Verification items for the finished model (mm, model axes). A direction names the side the tool comes from. Round coordinates to 2 decimals unless told otherwise and drop trailing zeros. Order: outer loops, then holes, each group sorted by start corner. A loop starts at its lowest first (then second) coordinate and runs counter-clockwise, first axis right, second up. Notation, with made-up numbers: (41.25, 32) -> (62.25, 32) arc R9 cw to (62.25, 39) -> close; hole circle Ø11 at (27, -32). An arc over 180 degrees is marked (long way). Put each result on its own line as item: value.
from build123d import *

# Parameters (mm, degrees)
BOSS_EXTRUDE2_DEPTH       = 8.5
BOSS_EXTRUDE2_DEPTH_BACK  = 8.5
M6_TAPPED_HOLE1_D         = 5
M3X0_5_TAPPED_HOLE1_D     = 2.5
M3X0_5_TAPPED_HOLE1_DEPTH = 7.5
M3X0_5_TAPPED_HOLE1_TIP   = 0.751075774


with BuildPart() as part:
    # Model → Boss-Extrude2 (new, two sides: drawn at the far end of the back side and taken through both)
    with BuildSketch(Plane.XY.offset(-BOSS_EXTRUDE2_DEPTH_BACK)):
        with BuildLine():
            Line((64.292892272, 21.792891862), (67.207107272, 24.707105862))
            ThreePointArc((67.207107272, 24.707105862), (67.423880138, 25.031529799), (67.500000272, 25.414213862))
            Line((67.500000272, 25.414213862), (67.500000272, 34.5857853))
            ThreePointArc((67.500000272, 34.5857853), (67.423879863, 34.968468589), (67.207107272, 35.292891862))
            Line((67.207107272, 35.292891862), (64.292892272, 38.207106862))
            ThreePointArc((64.292892272, 38.207106862), (63.96846972, 38.423879155), (63.585787272, 38.499999862))
            Line((63.585787272, 38.499999862), (62.500000272, 38.499999862))
            ThreePointArc((62.500000272, 38.499999862), (61.79289349, 38.207106644), (61.500000272, 37.499999862))
            Line((61.500000272, 37.499999862), (61.500000272, 34.899999862))
            Line((61.500000272, 34.899999862), (58.500000272, 34.899999862))
            Line((58.500000272, 34.899999862), (58.500000272, 25.099999862))
            Line((58.500000272, 25.099999862), (61.500000272, 25.099999862))
            Line((61.500000272, 25.099999862), (61.500000272, 22.499999862))
            ThreePointArc((61.500000272, 22.499999862), (61.79289349, 21.792893081), (62.500000272, 21.499999862))
            Line((62.500000272, 21.499999862), (63.585787272, 21.499999862))
            ThreePointArc((63.585787272, 21.499999862), (63.968469605, 21.576120108), (64.292892272, 21.792891862))
        make_face()
    extrude(amount=BOSS_EXTRUDE2_DEPTH + BOSS_EXTRUDE2_DEPTH_BACK)

    # M6 Tapped Hole1 (through all)
    with Locations(Plane.ZY.offset(-58.500000272)):
        with Locations((0, 29.999999862)):
            Hole(M6_TAPPED_HOLE1_D / 2)

    # M3x0.5 Tapped Hole1
    with Locations(Plane(origin=(0, 0, -8.5), x_dir=(-1, 0, 0), z_dir=(0, 0, -1))):
        with Locations((-64.461940205, 29.965764831)):
            Hole(M3X0_5_TAPPED_HOLE1_D / 2, depth=M3X0_5_TAPPED_HOLE1_DEPTH)
            with Locations((0, 0, -(M3X0_5_TAPPED_HOLE1_DEPTH + M3X0_5_TAPPED_HOLE1_TIP / 2))):  # 118° drill point
                Cone(0, M3X0_5_TAPPED_HOLE1_D / 2, M3X0_5_TAPPED_HOLE1_TIP, mode=Mode.SUBTRACT)


solid = part.part
Item 1: Tool access check on faces 4 (the flat face through (61.5, 24, 0)), 5 (the flat face through (65.8, 36.7, -0.1)), 6 (the flat face through (61.5, 36, 0)). Record the directions out of +Z, -Z, +X, -X, +Y, -Y that give a thin tool (end or side, any length) a straight path to the whole face; none if there is none.
Check sheet entries:
face 4: +Z, -Z, -X, -Y
face 5: +Z, -Z, +X, +Y
face 6: +Z, -Z, -X, +Y
Item 2: Gauge pin test, flat ends, axial feed: pin 1 Ø1.5 at (x, z) = (66.5, 5) entering from -Y; pin 2 Ø1.5 at (x, z) = (59.5, 1.5) entering from -Y; pin 3 Ø1.3 at (y, z) = (36.5, -0.5) entering from -X; pin 4 Ø3 at (y, z) = (30, 0) entering from -X. Record the tip position at first contact, or that the pin passes through.
Check sheet entries:
pin 1: stops at y = 23.25
pin 2: stops at y = 25.1
pin 3: stops at x = 61.5
pin 4: passes through
Item 3: Section check D-D on z = 4.75. Record the boundary of the cut face in (x, y), then the cut area to 3 significant figures.
Check sheet entries:
outline: (58.5, 25.1) -> (61.5, 25.1) -> (61.5, 22.5) arc R1 ccw to (62.5, 21.5) -> (63.59, 21.5) arc R1 ccw to (64.29, 21.79) -> (67.21, 24.71) arc R1 ccw to (67.5, 25.41) -> (67.5, 34.59) arc R1 ccw to (67.21, 35.29) -> (64.29, 38.21) arc R1 ccw to (63.59, 38.5) -> (62.5, 38.5) arc R1 ccw to (61.5, 37.5) -> (61.5, 34.9) -> (58.5, 34.9) -> close
area: 119 mm^2
Item 4: Release check for a two-part mould opening along Y. For faces 1 (the cylindrical face through (64.191, 28.745, -5.278)), 2 (the flat face through (65.7, 23.2, -0.1)), 3 (the flat face through (58.5, 32, -2)) record: +Y half, -Y half, draft (parallel to the pull), parting line (faces both ways), or undercut.
Check sheet entries:
face 1: undercut
face 2: -Y half
face 3: draft
Item 5: Section check C-C on x = 62.75. Record the boundary of the cut face in (y, z), then the cut area to 3 significant figures.
Check sheet entries:
outline: (21.5, -8.5) -> (38.5, -8.5) -> (38.5, 8.5) -> (21.5, 8.5) -> close; hole circle Ø5 at (30, 0)
area: 269 mm^2
Item 6: Section check A-A on z = 0. Record the boundary of the cut face in (x, y), then the cut area to 3 significant figures.
Check sheet entries:
outline: (58.5, 25.1) -> (61.5, 25.1) -> (61.5, 22.5) arc R1 ccw to (62.5, 21.5) -> (63.59, 21.5) arc R1 ccw to (64.29, 21.79) -> (67.21, 24.71) arc R1 ccw to (67.5, 25.41) -> (67.5, 27.5) -> (58.5, 27.5) -> close; (58.5, 32.5) -> (67.5, 32.5) -> (67.5, 34.59) arc R1 ccw to (67.21, 35.29) -> (64.29, 38.21) arc R1 ccw to (63.59, 38.5) -> (62.5, 38.5) arc R1 ccw to (61.5, 37.5) -> (61.5, 34.9) -> (58.5, 34.9) -> close
area: 73.6 mm^2
Item 7: Section check B-B on y = 31.5. Record the boundary of the cut face in (x, z).
Check sheet entries:
outline: (58.5, -8.5) -> (67.5, -8.5) -> (67.5, -2) -> (58.5, -2) -> close; (58.5, 2) -> (67.5, 2) -> (67.5, 8.5) -> (58.5, 8.5) -> close
Item 8: Material ranges on L1, parallel to X at y = 30, z = -3; L2, parallel to Z at x = 64.5, y = 30; L3, parallel to Y at x = 60.5, z = -7.5, recorded low to high. Write a range as [from, to].
Check sheet entries:
L1: x = [58.5, 63.21], [65.71, 67.5]
L2: z = [2.5, 8.5]
L3: y = [25.1, 34.9]
